Job drawing, mm, ordinate dimensions from the low corner. One solid piece. A direction names the side the tool comes from. Coordinates: 2 decimals unless noted, no trailing zeros. Order: outer loops, then holes, each group sorted by start corner. A loop starts at its lowest first (then second) coordinate and runs counter-clockwise, first axis right, second up. Notation, with made-up numbers: (34.25, 74.25) - (76.25, 74.25) arc R11 ccw to (76.25, 79.25) - close; hole circle Ø3 at (60, 47). An arc over 180 degrees is marked (long way). Return JSON: item names as keys, results as strings.
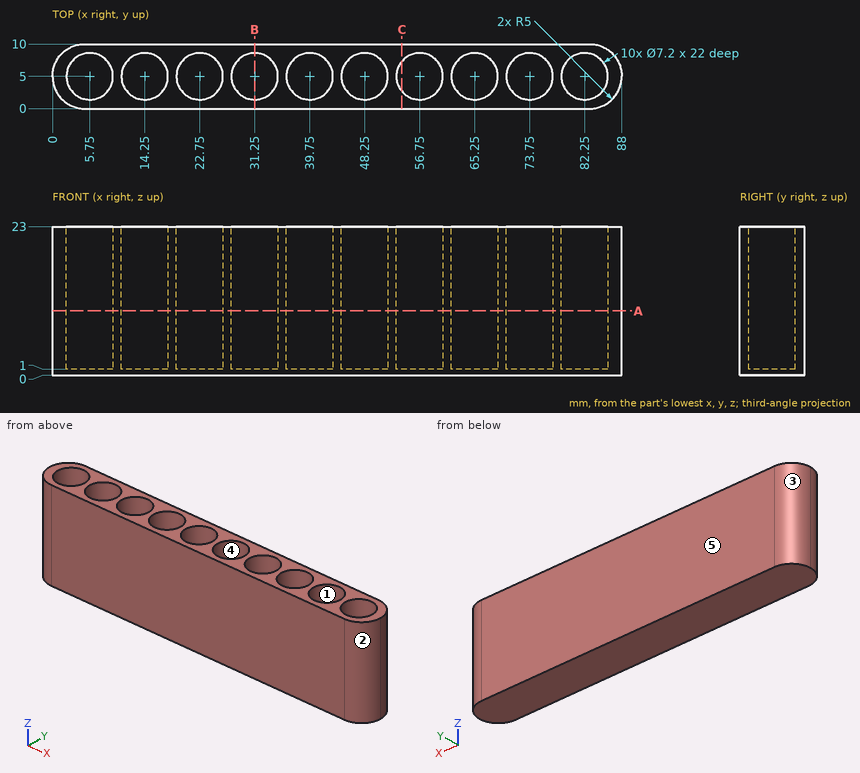
1. Drop flat-ended pins along their axis: pin 1 (6 mm diameter, centred on x = 5.5, y = 4.5, fed in from +Z); pin 2 (3 mm diameter, centred on x = 41.5, y = 6, fed in from -Z); pin 3 (6 mm diameter, centred on y = 8.5, z = 19, fed in from +X); pin 4 (4 mm diameter, centred on y = 1.5, z = 14, fed in from -X). Give the stop position or say it passes through.
Check values:
{"pin 1": "z = 1", "pin 2": "z = 0", "pin 3": "x = 87.97", "pin 4": "x = 0.23"}
2. Mould opens along Y. For the marked faces 1, 2 and 3 say: pulls with the +Y half, pulls with the -Y half, needs draft (parallel to the pull), parting line crosses it, or undercut.
Check values:
{"face 1": "undercut", "face 2": "pulls with the -Y half", "face 3": "pulls with the +Y half"}
3. Cut at C-C on x = 54. Give the cut face in (y, z).
Check values:
{"outline": "(0, 0) - (10, 0) - (10, 23) - (7.32, 23) - (7.32, 1) - (2.68, 1) - (2.68, 23) - (0, 23) - close"}
4. Probe L1, parallel to Y at x = 82.25, z = 12.75; L2, parallel to Y at x = 60, z = 9.25; L3, parallel to Z at x = 38.5, y = 6.5. List the from-to ranges inside material, lowest first.
Check values:
{"L1": "0 to 1.4, 8.6 to 10", "L2": "0 to 3.45, 6.55 to 10", "L3": "0 to 1"}
5. Cut at A-A on z = 10. State how many separate pieces and enclosed holes the cut face has, plus the area to 3 significant figures.
Check values:
{"separate pieces": "1", "enclosed holes": "10", "area": "451 mm²"}
6. Tool access for the marked faces 4 and 5: list every direction of +Z, -Z, +X, -X, +Y, -Y with a clear straight run to the whole face (end or side of a thin tool).
Check values:
{"face 4": "+Z", "face 5": "+Z, -Z, +X, -X, +Y"}
7. Cut at B-B on x = 31.25. Give the cut face in (y, z).
Check values:
{"outline": "(0, 0) - (10, 0) - (10, 23) - (8.6, 23) - (8.6, 1) - (1.4, 1) - (1.4, 23) - (0, 23) - close"}
